The drawing under review shows one solid part. Ordinate dimensions are in mm from its lowest x, y, z. Coordinates: 2 decimals unless noted, no trailing zeros. Write each loop counter-clockwise with the first axis right and the second up, starting at its lowest first coordinate (ties: lowest second). Pieces come first, ordered by that corner, then holes. Notation, with made-up numbers: (63, 65.25) - (82, 65.25) arc R12 cw to (82, 76.25) - close; hole circle Ø6 at (-0.75, 36). An arc over 180 degrees is marked (long way). Put each result on its own line as item: value. Start each with the question number.
Item 1: Consider section C-C on z = 6. Give the boundary of the cut face in (x, y), then the cut area to 3 significant figures.
Item 2: Consider section D-D on x = 2. Give the boundary of the cut face in (y, z).
Item 3: Consider section A-A on y = 11. Give the boundary of the cut face in (x, z), then the cut area to 4 significant figures.
Item 4: To check wall thickness, follow L1, parallel to Y at x = 11, z = 5.5; L2, parallel to Z at x = 14, y = 20; L3, parallel to X at y = 5.25, z = 8.25. State the ranges of each line that lie inside material, in increasing order. Write a range as [from, to].
Item 5: Mouldability with a two-part tool opening along X and no side actions: class the marked faces 1, 2 and 3 as pulls with the +X half, pulls with the -X half, needs draft (parallel to the pull), parting line crosses it, or undercut.
Item 6: For pin 1 (5 mm diameter, centred on x = 11, z = 7.5, fed in from -Y); pin 2 (4 mm diameter, centred on y = 5.5, z = 6.5, fed in from +X); pin 3 (2 mm diameter, centred on y = 9.5, z = 8.5, fed in from -X); pin 4 (5 mm diameter, centred on x = 17.5, y = 19, fed in from -Z), all flat-tipped, find the tip position at first contact; note any pin that passes through.
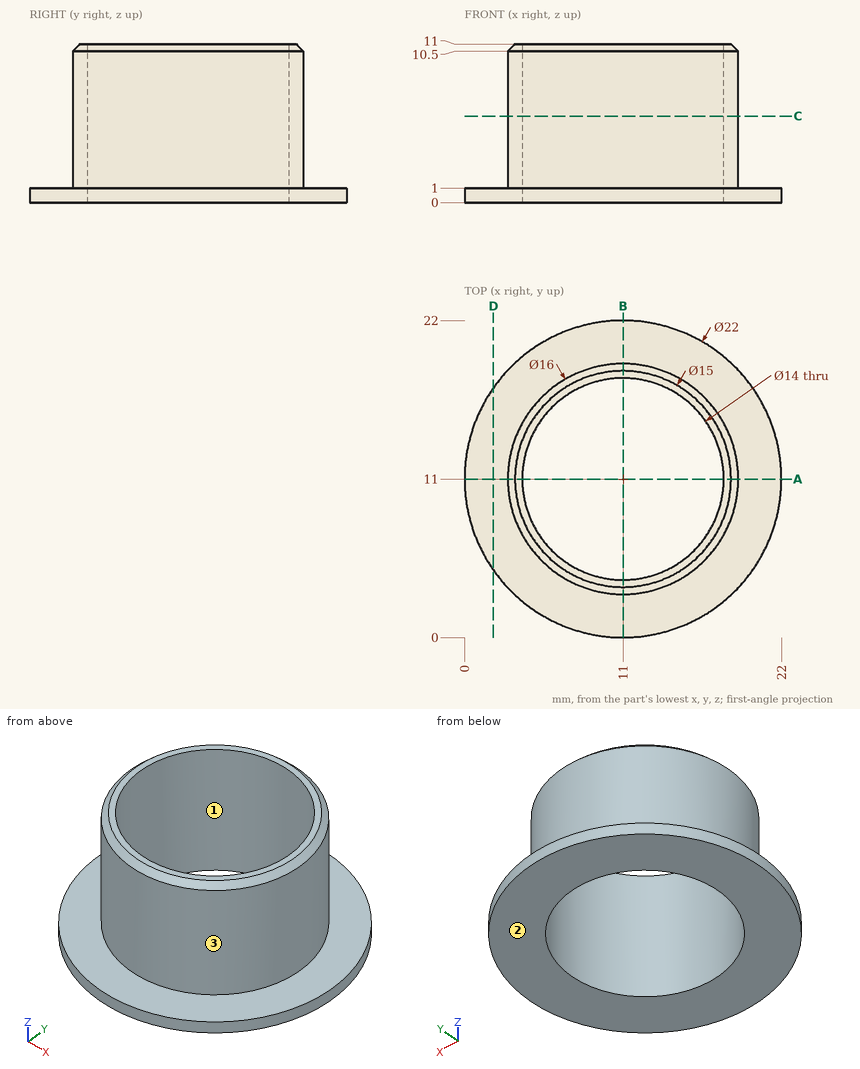
Report:
1. outline: circle Ø16 at (11, 11); hole circle Ø14 at (11, 11)
1. area: 47.1 mm²
2. outline: (4.68, 0) - (17.32, 0) - (17.32, 1) - (4.68, 1) - close
3. outline: (0, 0) - (4, 0) - (4, 11) - (3.5, 11) - (3, 10.5) - (3, 1) - (0, 1) - close; (18, 0) - (22, 0) - (22, 1) - (19, 1) - (19, 10.5) - (18.5, 11) - (18, 11) - close
3. area: 27.75 mm²
4. L1: [3, 4], [18, 19]
4. L2: [0, 1]
4. L3: [5.44, 7.01], [14.99, 16.56]
5. face 1: undercut
5. face 2: needs draft
5. face 3: parting line crosses it
6. pin 1: y = 3
6. pin 2: x = 18.19
6. pin 3: x = 3.02
6. pin 4: z = 0
